Can you work these out from the model? Positions are in its coordinate system, mm. Face numbers are marked on the shaded views. Give positions to 0.01 mm unless a question says otherwise; leave off trailing zeros. Order: outer loops, then holes, each group sorted by start corner. A loop starts at its lowest first (then second) coordinate and runs counter-clockwise, first axis right, second up.
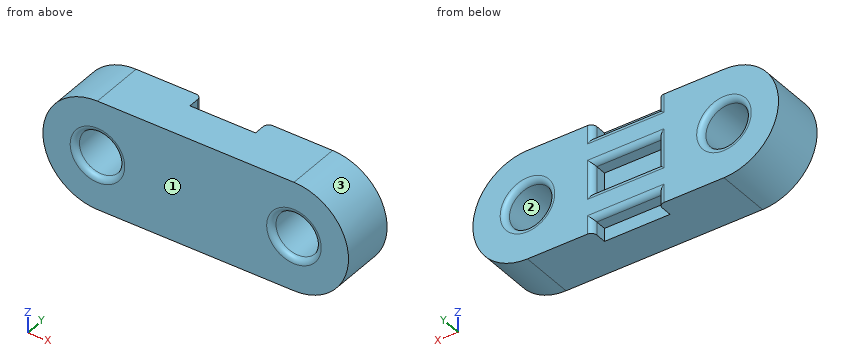
```python
from build123d import *

# Parameters (mm, degrees)
BOSS_EXTRUDE1_DEPTH = 5
SCREW_HOLES_R       = 2
CUT_EXTRUDE1_DEPTH  = 5
FILLET2_R           = 0.5
BELT_CUT_OUTS_W     = 6
BELT_CUT_OUTS_H     = 1.2
BELT_CUT_OUTS_H_2   = 2.6
CUT_EXTRUDE2_DEPTH  = 1.5
FILLET3_R           = 0.5


with BuildPart() as part:
    # Belt Clamp → Boss-Extrude1 (new body)
    with BuildSketch(Plane(origin=(0, 0, 0), x_dir=(1, 0, 0), z_dir=(0, 1, 0))):
        with BuildLine():
            Line((-18, 10), (0, 10))
            ThreePointArc((0, 10), (5, 5), (0, 0))
            Line((0, 0), (-18, 0))
            ThreePointArc((-18, 0), (-23, 5), (-18, 10))
        make_face()
    extrude(amount=BOSS_EXTRUDE1_DEPTH)

    # Screw Holes → Cut-Extrude1 (cut)
    with BuildSketch(Plane.XZ):
        with Locations(Location((-18, -5, 0), (0, 0, 270))):
            Circle(SCREW_HOLES_R)
        with Locations(Location((0, -5, 0), (0, 0, 270))):
            Circle(SCREW_HOLES_R)
    extrude(amount=-CUT_EXTRUDE1_DEPTH, mode=Mode.SUBTRACT)

    # Fillet2
    fillet2_edges = [part.edges().sort_by_distance(p)[0] for p in [
        (-18, 0, -3),
        (-18, 5, -3),
        (0, 0, -3),
        (0, 5, -3),
    ]]
    fillet(fillet2_edges, radius=FILLET2_R)

    # Belt cut outs → Cut-Extrude2 (cut)
    with BuildSketch(Plane(origin=(0, 5, 0), x_dir=(1, 0, 0), z_dir=(0, 1, 0))):
        with Locations((-9, 0.6)):
            Rectangle(BELT_CUT_OUTS_W, BELT_CUT_OUTS_H)
        with Locations((-9, 5)):
            Rectangle(BELT_CUT_OUTS_W, BELT_CUT_OUTS_H_2)
        with Locations((-9, 9.4)):
            Rectangle(BELT_CUT_OUTS_W, BELT_CUT_OUTS_H)
    extrude(amount=-CUT_EXTRUDE2_DEPTH, mode=Mode.SUBTRACT)

    # Fillet3
    fillet3_edges = [part.edges().sort_by_distance(p)[0] for p in [
        (-12, 5, -0.6),
        (-6, 5, -0.6),
        (-9, 5, -1.2),
        (-12, 5, -9.4),
        (-9, 5, -8.8),
        (-6, 5, -9.4),
        (-12, 5, -5),
        (-9, 5, -3.7),
        (-6, 5, -5),
        (-9, 5, -6.3),
    ]]
    fillet(fillet3_edges, radius=FILLET3_R)


solid = part.part
```
1) Suppose I cut it at A-A (z = -5). Please give me the cut outline in (x, y).
2) I'm going to push flat-ended pins straight in: pin 1 Ø1.1 at (y, z) = (4, -0.5) entering from -X; pin 2 Ø6 at (x, z) = (-16, -2.5) entering from -Y; pin 3 Ø0.8 at (x, y) = (-8.5, 4) entering from +Z; pin 4 Ø0.5 at (y, z) = (4, -9.5) entering from -X. Where does each tip first touch, or does it pass through?
3) We'd pull the mould along X, two halves only. Please class the marked faces 1, 2 and 3: +X half, -X half, draft (parallel to the pull), parting line (faces both ways), or undercut.
4) Suppose I cut it at B-B (y = 2.05). Please give me the cut outline in (x, z), and give its area (3 significant figures).
5) If I drill on line 1 (X direction, y = 1.4, z = -5); line 2 (X direction, y = 3.6, z = -5); line 3 (X direction, y = 2.25, z = -6), over which ranges is the centre line in solid material (lowest first)?
Results:
1. outline: (-23, 0) - (-20.5, 0) arc R0.5 ccw to (-20, 0.5) - (-20, 4.5) arc R0.5 ccw to (-20.5, 5) - (-23, 5) - close; (-16, 0.5) arc R0.5 ccw to (-15.5, 0) - (-2.5, 0) arc R0.5 ccw to (-2, 0.5) - (-2, 4.5) arc R0.5 ccw to (-2.5, 5) - (-5.5, 5) arc R0.5 ccw to (-6, 4.5) - (-6, 3.5) - (-12, 3.5) - (-12, 4.5) arc R0.5 ccw to (-12.5, 5) - (-15.5, 5) arc R0.5 ccw to (-16, 4.5) - close; (2, 0.5) arc R0.5 ccw to (2.5, 0) - (5, 0) - (5, 5) - (2.5, 5) arc R0.5 ccw to (2, 4.5) - close
2. pin 1: stops at x = -21.07
2. pin 2: stops at y = 0
2. pin 3: stops at z = -1.2
2. pin 4: stops at x = -20.63
3. face 1: draft
3. face 2: undercut
3. face 3: +X half
4. outline: (-18, -10) - (0, -10) arc R5 ccw to (0, 0) - (-18, 0) arc R5 ccw to start; hole circle Ø4 at (-18, -5); hole circle Ø4 at (0, -5)
4. area: 233 mm2
5. line 1: x = -23 to -20, -16 to -2, 2 to 5
5. line 2: x = -23 to -20, -16 to -12, -6 to -2, 2 to 5
5. line 3: x = -22.9 to -19.73, -16.27 to -1.73, 1.73 to 4.9
